```python
from build123d import *

# Parameters (mm, degrees)
SKETCH1_R           = 18
SKETCH1_R_2         = 12
BOSS_EXTRUDE1_DEPTH = 10
SKETCH3_R           = 14.2
CUT_EXTRUDE1_DEPTH  = 1.75
SKETCH5_R           = 14.25
SKETCH5_R_2         = 12
BOSS_EXTRUDE2_DEPTH = 10
CHAMFER1_SIZE       = 2


with BuildPart() as part:
    # Sketch1 → Boss-Extrude1 (new body)
    with BuildSketch(Plane.XY):
        Circle(SKETCH1_R)
        Circle(SKETCH1_R_2, mode=Mode.SUBTRACT)
    extrude(amount=BOSS_EXTRUDE1_DEPTH)

    # Sketch3 → Cut-Extrude1 (cut)
    with BuildSketch(Plane.XY):
        Circle(SKETCH3_R)
    extrude(amount=CUT_EXTRUDE1_DEPTH, mode=Mode.SUBTRACT)

    # Sketch5 → Boss-Extrude2 (add)
    with BuildSketch(Plane.XY.offset(10)):
        Circle(SKETCH5_R)
        Circle(SKETCH5_R_2, mode=Mode.SUBTRACT)
    extrude(amount=BOSS_EXTRUDE2_DEPTH)

    # Chamfer1
    chamfer1_edges = [part.edges().sort_by_distance(p)[0] for p in [
        (-14.25, 0, 10),
    ]]
    chamfer(chamfer1_edges, length=CHAMFER1_SIZE)


solid = part.part
```
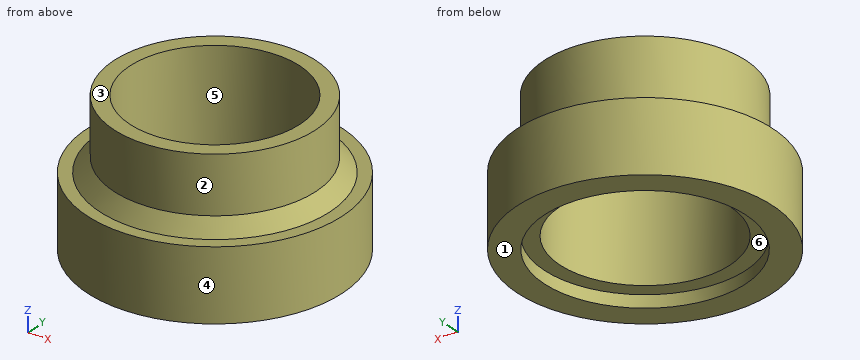
Design review of the part built by this model. Coordinates are the model's own, in mm. Face numbers are marked on the shaded views. A direction names the side the tool comes from. Round coordinates to 2 decimals unless told otherwise and drop trailing zeros. Write each loop counter-clockwise with the first axis right and the second up, starting at its lowest first coordinate (ties: lowest second). Pieces come first, ordered by that corner, then holes. Notation, with made-up numbers: (13.25, 14) -> (62.25, 14) arc R25 ccw to (62.25, 33) -> close; hole circle Ø4 at (57.25, 86). An arc over 180 degrees is marked (long way). Write item = value, one per line. Start each with the question number.
1) Mouldability with a two-part tool opening along Y and no side actions: class the marked faces 3, 4, 5 and 6 as +Y half, -Y half, draft (parallel to the pull), parting line (faces both ways), or undercut.
2) Take a section at A-A, the plane y = 0. State the section outline as (x, z) points.
3) Tool access review of the marked faces 1 and 2: name each direction out of +Z, -Z, +X, -X, +Y, -Y from which nothing blocks a thin tool from reaching the whole face with its end or side.
4) Wall thickness on probe 1 along Y at (x, z) = (0, 0.65); probe 2 along Y at (x, z) = (0, 14); probe 3 along Z at (x, y) = (13.5, -9.5): over which ranges is each line inside the solid? List them lowest first. Write a range as from..to.
5) Take a section at C-C, the plane z = 5.5. State the section outline as (x, y) points.
6) Clearance check with flat-ended pins moving along their axes: pin 1 (5 mm diameter, centred on x = -5, z = 9, fed in from -Y); pin 2 (10 mm diameter, centred on x = 2, y = 6.5, fed in from +Z); pin 3 (2 mm diameter, centred on y = 13, z = 16, fed in from +X); pin 4 (5 mm diameter, centred on y = 3, z = 4.5, fed in from +X). State where each tip first meets the part, or that it passes through.
7) Take a section at D-D, the plane z = 14.5. State the section outline as (x, y) points, plus the area to 3 significant figures.
Results list:
q1.face_3 = draft
q1.face_4 = parting line
q1.face_5 = undercut
q1.face_6 = undercut
q2.outline = (-18, 0) -> (-14.2, 0) -> (-14.2, 1.75) -> (-12, 1.75) -> (-12, 20) -> (-14.25, 20) -> (-14.25, 12) -> (-16.25, 10) -> (-18, 10) -> close; (12, 1.75) -> (14.2, 1.75) -> (14.2, 0) -> (18, 0) -> (18, 10) -> (16.25, 10) -> (14.25, 12) -> (14.25, 20) -> (12, 20) -> close
q3.face_1 = -Z, +X, -X, +Y, -Y
q3.face_2 = +Z
q4.probe_1 = -18..-14.2, 14.2..18
q4.probe_2 = -14.25..-12, 12..14.25
q4.probe_3 = 0..10
q5.outline = circle Ø36 at (0, 0); hole circle Ø24 at (0, 0)
q6.pin_1 = -17.83
q6.pin_2 = through
q6.pin_3 = 7.69
q6.pin_4 = 17.99
q7.outline = circle Ø28.5 at (0, 0); hole circle Ø24 at (0, 0)
q7.area = 186 mm²
